Source: CAD feature listing. Evaluate the final solid. Frame: model axes, mm. A direction names the side the tool comes from. Coordinates: 2 decimals unless noted, no trailing zeros. Loops run counter-clockwise (first coordinate to the right, second up) from the corner with the lowest first, then second, coordinate; pieces in that order, holes last.
from build123d import *

# Parameters (mm, degrees)
RESSALTO_EXTRUS_O1_DEPTH                      = 20
BROCA_DE_ROSQUEAR_PARA_HELICOIDE_M31_AT_COUNT = 2
BROCA_DE_ROSQUEAR_PARA_HELICOIDE_M31_AT_PITCH = 13.431658115
BROCA_DE_ROSQUEAR_PARA_HELICOIDE_M31_2_COUNT  = 2
BROCA_DE_ROSQUEAR_PARA_HELICOIDE_M31_2_PITCH  = 38.822958194
BROCA_DE_ROSQUEAR_PARA_HELICOIDE_M31_3_COUNT  = 2
BROCA_DE_ROSQUEAR_PARA_HELICOIDE_M31_3_PITCH  = 41.080792624
BROCA_DE_ROSQUEAR_PARA_HELICOIDE_M32_D        = 3.5
BROCA_DE_ROSQUEAR_PARA_HELICOIDE_M32_DEPTH    = 10
BROCA_DE_ROSQUEAR_PARA_HELICOIDE_M32_TIP      = 1.051506083


with BuildPart() as part:
    # Esboço1 → Ressalto-extrusão1 (new body)
    with BuildSketch(Plane.XY):
        Polygon((-29.202088452, -18.454545455), (-29.202088452, -16.454545455), (-24.656633907, -16.454545455), (-24.656633907, 19.545454545), (9.343366093, 19.545454545), (9.343366093, -17), (14.797911548, -17), (14.797911548, -19), (7.343366093, -19), (7.343366093, 17.545454545), (-22.656633907, 17.545454545), (-22.656633907, -16.454545455), (-22.656633907, -18.454545455), align=None)
    extrude(amount=RESSALTO_EXTRUS_O1_DEPTH)

    # Esboço3 → Broca de rosquear para helicoide M31 (revolve, cut)
    with BuildSketch(Plane(origin=(12.189799686, -17, 3.965200957), x_dir=(0, 0, 1), z_dir=(1, 0, 0))):
        Polygon((0, 0), (0, 11.051506083), (1.75, 10), (1.75, 0), align=None)
    broca_de_rosquear_para_helicoide_m31 = revolve(axis=Axis((12.189799686, -10.65, 3.965200957), (0, -1, 0)), mode=Mode.SUBTRACT)

    # Broca de rosquear para helicoide M31 at: Broca de rosquear para helicoide M31 ×2
    with Locations(*[(0, 0, i * BROCA_DE_ROSQUEAR_PARA_HELICOIDE_M31_AT_PITCH) for i in range(1, BROCA_DE_ROSQUEAR_PARA_HELICOIDE_M31_AT_COUNT)]):
        add(broca_de_rosquear_para_helicoide_m31, mode=Mode.SUBTRACT)

    # Broca de rosquear para helicoide M31 2: Broca de rosquear para helicoide M31 ×2
    with Locations(*[(-i * BROCA_DE_ROSQUEAR_PARA_HELICOIDE_M31_2_PITCH, 0, 0) for i in range(1, BROCA_DE_ROSQUEAR_PARA_HELICOIDE_M31_2_COUNT)]):
        add(broca_de_rosquear_para_helicoide_m31, mode=Mode.SUBTRACT)

    # Broca de rosquear para helicoide M31 3: Broca de rosquear para helicoide M31 ×2
    with Locations(*[Vector(-0.9450391707113346, 0, 0.3269571314732758) * (i * BROCA_DE_ROSQUEAR_PARA_HELICOIDE_M31_3_PITCH) for i in range(1, BROCA_DE_ROSQUEAR_PARA_HELICOIDE_M31_3_COUNT)]):
        add(broca_de_rosquear_para_helicoide_m31, mode=Mode.SUBTRACT)

    # Broca de rosquear para helicoide M32
    with Locations(Plane(origin=(0, -16.454545455, 0), x_dir=(1, 0, 0), z_dir=(0, 1, 0))):
        with Locations((-26.864375338, -17.411313342), (-26.864375338, -4.228770119)):
            Hole(BROCA_DE_ROSQUEAR_PARA_HELICOIDE_M32_D / 2, depth=BROCA_DE_ROSQUEAR_PARA_HELICOIDE_M32_DEPTH)
            with Locations((0, 0, -(BROCA_DE_ROSQUEAR_PARA_HELICOIDE_M32_DEPTH + BROCA_DE_ROSQUEAR_PARA_HELICOIDE_M32_TIP / 2))):  # 118° drill point
                Cone(0, BROCA_DE_ROSQUEAR_PARA_HELICOIDE_M32_D / 2, BROCA_DE_ROSQUEAR_PARA_HELICOIDE_M32_TIP, mode=Mode.SUBTRACT)


solid = part.part
Q1. Access query for faces 1 (the flat face through (7.343, -1, 10)), 2 (the flat face through (-26, -18.455, 10)), 3 (the flat face through (12, -17, 10)), 4 (the cylindrical face through (-24.89, -17.72, 17.25)). Directions: +Z, -Z, +X, -X, +Y, -Y. A direction counts if a zero-diameter tool reaches every point of the face in a straight line with its end or side. Return the directions, or none.
Q2. Section D-D, the plane x = -8. Return the cut outline in (y, z).
Q3. Section A-A, the plane y = 16.5. Return the cut outline in (x, z), plus the area to 3 significant figures.
Q4. Section C-C, the plane z = 1.5. Return the cut outline in (x, y), plus the area to 3 significant figures.
Q5. Draft query along Z for faces 5 (the cylindrical face through (-27.672, -17.246, 5.781)), 6 (the flat face through (-22.657, -1, 10)), 7 (the flat face through (8, 2, 20)). Return one class per face: +Z half, -Z half, draft (parallel to the pull), parting line (faces both ways), or undercut.
Q6. Contact query for flat-ended pins moving along their axis: pin 1 Ø12 at (x, z) = (-24.5, 3) entering from -Y; pin 2 Ø1.4 at (x, z) = (-27.5, 10.5) entering from +Y; pin 3 Ø3 at (x, z) = (12.19, 3.97) entering from +Y; pin 4 Ø6 at (y, z) = (-5, 9.5) entering from +X. Output: stop coordinate, or through.
Q7. Line query: line 1 along X through (y, z) = (-0.5, 6); line 2 along Y through (x, z) = (-11.5, 6.5); line 3 along Y through (x, z) = (-27, 1). Output: solid intervals per line, ascending.
Q8. Section B-B, the plane z = 16.25. Return the cut outline in (x, y), plus the area to 3 significant figures.
Derived:
1. face 1: +Z, -Z, -Y
1. face 2: +Z, -Z, -X, -Y
1. face 3: +Z, -Z, +X, +Y
1. face 4: -Y
2. outline: (17.55, 0) - (19.55, 0) - (19.55, 20) - (17.55, 20) - close
3. outline: (-24.66, 0) - (-22.66, 0) - (-22.66, 20) - (-24.66, 20) - close; (7.34, 0) - (9.34, 0) - (9.34, 20) - (7.34, 20) - close
3. area: 80.0 mm2
4. outline: (-29.2, -18.45) - (-22.66, -18.45) - (-22.66, 17.55) - (7.34, 17.55) - (7.34, -19) - (14.8, -19) - (14.8, -17) - (9.34, -17) - (9.34, 19.55) - (-24.66, 19.55) - (-24.66, -16.45) - (-29.2, -16.45) - close
4. area: 233 mm2
5. face 5: undercut
5. face 6: draft
5. face 7: +Z half
6. pin 1: stops at y = -18.45
6. pin 2: stops at y = -16.45
6. pin 3: passes through
6. pin 4: stops at x = 9.34
7. line 1: x = -24.66 to -22.66, 7.34 to 9.34
7. line 2: y = 17.55 to 19.55
7. line 3: y = -18.45 to -16.45
8. outline: (-29.2, -18.45) - (-28.17, -18.45) - (-28.17, -16.45) - (-29.2, -16.45) - close; (-25.56, -17) - (-25.31, -17) - (-25.31, -18.45) - (-22.66, -18.45) - (-22.66, 17.55) - (7.34, 17.55) - (7.34, -19) - (10.87, -19) - (10.87, -17) - (9.34, -17) - (9.34, 19.55) - (-24.66, 19.55) - (-24.66, -16.45) - (-25.56, -16.45) - close; (13.51, -19) - (14.8, -19) - (14.8, -17) - (13.51, -17) - close
8. area: 222 mm2
